```python
from build123d import *

# Parameters (mm, degrees)
SKETCH3_R                = 6.35
SKETCH3_R_2              = 2.1082
BOSS_EXTRUDE1_DEPTH      = 3.175
BOSS_EXTRUDE1_DEPTH_BACK = 3.175
CHAMFER1_SIZE            = 0.508


with BuildPart() as part:
    # Sketch3 → Boss-Extrude1 (new body, two sides)
    with BuildSketch(Plane.XY) as boss_extrude1_sk:
        Circle(SKETCH3_R)
        Circle(SKETCH3_R_2, mode=Mode.SUBTRACT)
    extrude(amount=BOSS_EXTRUDE1_DEPTH)
    extrude(boss_extrude1_sk.sketch, amount=-BOSS_EXTRUDE1_DEPTH_BACK)

    # Chamfer1
    chamfer1_edges = [part.edges().sort_by_distance(p)[0] for p in [
        (-6.35, 0, -3.175),
        (-2.1082, 0, -3.175),
        (-6.35, 0, 3.175),
        (-2.1082, 0, 3.175),
    ]]
    chamfer(chamfer1_edges, length=CHAMFER1_SIZE)


solid = part.part
```
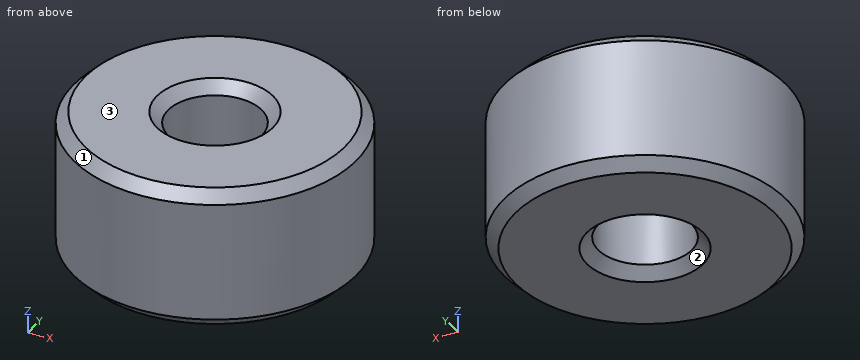
Input: part model. Units: mm. Frame: model coordinates. Face numbers are marked on the shaded views. Round coordinates to 2 decimals unless told otherwise and drop trailing zeros. Write each loop counter-clockwise with the first axis right and the second up, starting at its lowest first coordinate (ties: lowest second). Pieces come first, ordered by that corner, then holes. Notation, with made-up numbers: (-15, 83.5) - (26, 83.5) arc R35 ccw to (26, 115.5) - close; hole circle Ø1 at (77.5, 80.5). An arc over 180 degrees is marked (long way). Write item = value, one per line.
(1) Pull-direction query (X, two-part tool) for the marked faces 1, 2 and 3; classes: +X half, -X half, draft (parallel to the pull), parting line (faces both ways), or undercut.
Geometry check:
face_1 = parting line
face_2 = undercut
face_3 = draft
(2) Contact query for flat-ended pins moving along their axis: pin 1 Ø1.5 at (y, z) = (-3.5, -1.5) entering from -X; pin 2 Ø1.5 at (y, z) = (2, -0.5) entering from -X. Output: stop coordinate, or through.
Geometry check:
pin_1 = -5.72
pin_2 = -6.23
(3) Section query A-A on x = 0. Output: boundary loops of the cut face in (y, z) (3 decimals), then the cut area to 3 significant figures.
Geometry check:
outline = (-6.35, -2.667) - (-5.842, -3.175) - (-2.616, -3.175) - (-2.108, -2.667) - (-2.108, 2.667) - (-2.616, 3.175) - (-5.842, 3.175) - (-6.35, 2.667) - close; (2.108, -2.667) - (2.616, -3.175) - (5.842, -3.175) - (6.35, -2.667) - (6.35, 2.667) - (5.842, 3.175) - (2.616, 3.175) - (2.108, 2.667) - close
area = 52.8 mm^2
(4) Section query C-C on z = 2. Output: boundary loops of the cut face in (x, y).
Geometry check:
outline = circle Ø12.7 at (0, 0); hole circle Ø4.22 at (0, 0)
(5) Material intervals for probe 1 along Y at (x, z) = (0, -1.5); probe 2 along X at (y, z) = (-1, -2.75); probe 3 along X at (y, z) = (3, 1.5), sorted ascending.
Geometry check:
probe_1 = -6.35 to -2.11, 2.11 to 6.35
probe_2 = -6.19 to -1.95, 1.95 to 6.19
probe_3 = -5.6 to 5.6
